The listing builds one solid part. Answer for the finished solid, in the listing's coordinates (mm). Face numbers are marked on the shaded views. Coordinates: 2 decimals unless noted, no trailing zeros. Order: outer loops, then holes, each group sorted by start corner. A loop starts at its lowest first (then second) coordinate and runs counter-clockwise, first axis right, second up.
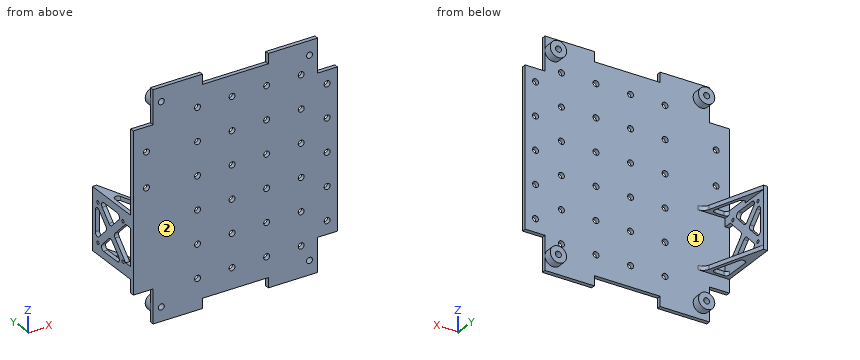
```python
from build123d import *

# Parameters (mm, degrees)
SKETCH1_R            = 2.286
MAIN_BODY_DEPTH      = 3.175
SKETCH34_W           = 7.62
SKETCH34_H           = 50.8
BOSS_EXTRUDE3_DEPTH  = 3.175
SKETCH35_R           = 6.28142
SKETCH35_R_2         = 2.286
BOSS_EXTRUDE4_DEPTH  = 6.35
SKETCH37_W           = 3.175
SKETCH37_H           = 47.625
BOSS_EXTRUDE5_DEPTH  = 45.72
SKETCH40_R           = 1.25
CUT_EXTRUDE3_DEPTH   = 3.175
CUT_EXTRUDE6_REACH   = 188.437
SKETCH48_W           = 28.575
SKETCH48_H           = 6.0825
SKETCH49_R           = 2.286
CUT_EXTRUDE7_DEPTH   = 126.930282399
EXTRUDE_THIN1_DEPTH  = 3.175
FILLET1_R            = 2.54
FILLET2_R            = 6.35
FILLET1_OF_MIRROR2_R = 2.54
FILLET2_OF_MIRROR2_R = 6.35
SKETCH50_R           = 2.286
CUT_EXTRUDE8_DEPTH   = 126.930282399


with BuildPart() as part:
    # Sketch1 → Main Body (new body)
    with BuildSketch(Plane(origin=(0, 0, 0), x_dir=(1, 0, 0), z_dir=(0, 1, 0))):
        Polygon((-25.4, 86.995), (-63.43142, 86.995), (-63.43142, 60.96), (-78.74, 60.96), (-78.74, 25.4), (-71.12, 25.4), (-71.12, -25.4), (-78.74, -25.4), (-78.74, -60.96), (-63.43142, -60.96), (-63.43142, -86.995), (-25.4, -86.995), (-25.4, -79.375), (25.4, -79.375), (25.4, -86.995), (63.43142, -86.995), (63.43142, -60.96), (78.74, -60.96), (78.74, -25.4), (71.12, -25.4), (71.12, 25.4), (78.74, 25.4), (78.74, 60.96), (63.43142, 60.96), (63.43142, 86.995), (25.4, 86.995), (25.4, 79.375), (-25.4, 79.375), align=None)
        with Locations(Location((-57.15, 76.2, 0), (0, 0, 270))):
            Circle(SKETCH1_R, mode=Mode.SUBTRACT)
        with Locations(Location((57.15, 76.2, 0), (0, 0, 270))):
            Circle(SKETCH1_R, mode=Mode.SUBTRACT)
        with Locations(Location((57.15, -76.2, 0), (0, 0, 270))):
            Circle(SKETCH1_R, mode=Mode.SUBTRACT)
        with Locations(Location((-57.15, -76.2, 0), (0, 0, 270))):
            Circle(SKETCH1_R, mode=Mode.SUBTRACT)
    extrude(amount=MAIN_BODY_DEPTH)

    # Sketch34 → Boss-Extrude3 (add)
    with BuildSketch(Plane(origin=(0, 3.175, 0), x_dir=(1, 0, 0), z_dir=(0, 1, 0))):
        with Locations((-74.93, 0)):
            Rectangle(SKETCH34_W, SKETCH34_H)
        with Locations((74.93, 0)):
            Rectangle(SKETCH34_W, SKETCH34_H)
    extrude(amount=-BOSS_EXTRUDE3_DEPTH)

    # Sketch35 → Boss-Extrude4 (add)
    # profile 1 of 4: a face of its own
    with BuildSketch(Plane(origin=(0, 3.175, 0), x_dir=(1, 0, 0), z_dir=(0, 1, 0))):
        with Locations((57.15, 76.2)):
            Circle(SKETCH35_R)
        with Locations(Location((57.15, 76.2, 0), (0, 0, 270))):
            Circle(SKETCH35_R_2, mode=Mode.SUBTRACT)
    # profile 2 of 4: a face of its own
    with BuildSketch(Plane(origin=(0, 3.175, 0), x_dir=(1, 0, 0), z_dir=(0, 1, 0))):
        with Locations((57.15, -76.2)):
            Circle(SKETCH35_R)
        with Locations(Location((57.15, -76.2, 0), (0, 0, 270))):
            Circle(SKETCH35_R_2, mode=Mode.SUBTRACT)
    # profile 3 of 4: a face of its own
    with BuildSketch(Plane(origin=(0, 3.175, 0), x_dir=(1, 0, 0), z_dir=(0, 1, 0))):
        with Locations(Location((-57.15, -76.2, 0), (0, 0, 180))):
            Circle(SKETCH35_R)
        with Locations(Location((-57.15, -76.2, 0), (0, 0, 270))):
            Circle(SKETCH35_R_2, mode=Mode.SUBTRACT)
    # profile 4 of 4: a face of its own
    with BuildSketch(Plane(origin=(0, 3.175, 0), x_dir=(1, 0, 0), z_dir=(0, 1, 0))):
        with Locations(Location((-57.15, 76.2, 0), (0, 0, 180))):
            Circle(SKETCH35_R)
        with Locations(Location((-57.15, 76.2, 0), (0, 0, 270))):
            Circle(SKETCH35_R_2, mode=Mode.SUBTRACT)
    extrude(amount=BOSS_EXTRUDE4_DEPTH)

    # Sketch37 → Boss-Extrude5 (add)
    with BuildSketch(Plane(origin=(0, 3.175, 0), x_dir=(1, 0, 0), z_dir=(0, 1, 0))):
        with Locations((-77.1525, 26.9875)):
            Rectangle(SKETCH37_W, SKETCH37_H)
    extrude(amount=BOSS_EXTRUDE5_DEPTH)

    # Sketch40 → Cut-Extrude3 (cut)
    with BuildSketch(Plane.ZY.offset(78.74)):
        with Locations((-41.9875, 42.355)):
            Circle(SKETCH40_R)
        with Locations((-11.9875, 42.355)):
            Circle(SKETCH40_R)
        with Locations((-11.9875, 12.355)):
            Circle(SKETCH40_R)
        with Locations((-41.9875, 12.355)):
            Circle(SKETCH40_R)
        with BuildLine():
            Line((-35.142897552, 45.4525), (-18.832102448, 45.4525))
            ThreePointArc((-18.832102448, 45.4525), (-16.485448436, 43.884515918), (-17.036051224, 41.116448776))
            Line((-17.036051224, 41.116448776), (-25.191448776, 32.961051224))
            ThreePointArc((-25.191448776, 32.961051224), (-26.9875, 32.217102448), (-28.783551224, 32.961051224))
            Line((-28.783551224, 32.961051224), (-36.938948776, 41.116448776))
            ThreePointArc((-36.938948776, 41.116448776), (-37.489551564, 43.884515918), (-35.142897552, 45.4525))
        make_face()
        with BuildLine():
            Line((-21.381448776, 29.151051224), (-13.226051224, 37.306448776))
            ThreePointArc((-13.226051224, 37.306448776), (-10.457984082, 37.857051564), (-8.89, 35.510397552))
            Line((-8.89, 35.510397552), (-8.89, 19.199602448))
            ThreePointArc((-8.89, 19.199602448), (-10.457984082, 16.852948436), (-13.226051224, 17.403551224))
            Line((-13.226051224, 17.403551224), (-21.381448776, 25.558948776))
            ThreePointArc((-21.381448776, 25.558948776), (-22.125397552, 27.355), (-21.381448776, 29.151051224))
        make_face()
        with BuildLine():
            Line((-25.191448776, 21.748948776), (-12.7, 9.2575))
            Line((-12.7, 9.2575), (-41.275, 9.2575))
            Line((-41.275, 9.2575), (-28.783551224, 21.748948776))
            ThreePointArc((-28.783551224, 21.748948776), (-26.9875, 22.492897552), (-25.191448776, 21.748948776))
        make_face()
        with BuildLine():
            Line((-32.593551224, 25.558948776), (-40.748948776, 17.403551224))
            ThreePointArc((-40.748948776, 17.403551224), (-43.517015918, 16.852948436), (-45.085, 19.199602448))
            Line((-45.085, 19.199602448), (-45.085, 35.510397552))
            ThreePointArc((-45.085, 35.510397552), (-43.517015918, 37.857051564), (-40.748948776, 37.306448776))
            Line((-40.748948776, 37.306448776), (-32.593551224, 29.151051224))
            ThreePointArc((-32.593551224, 29.151051224), (-31.849602448, 27.355), (-32.593551224, 25.558948776))
        make_face()
    extrude(amount=-CUT_EXTRUDE3_DEPTH, mode=Mode.SUBTRACT)

    # Sketch48 → Cut-Extrude6 (cut, up to next)
    with BuildSketch(Plane.ZY.offset(78.74), mode=Mode.PRIVATE) as cut_extrude6_sk1:
        with Locations((-26.9875, 6.21625)):
            Rectangle(SKETCH48_W, SKETCH48_H)
    cut_extrude6_tool1 = extrude(cut_extrude6_sk1.sketch, amount=-CUT_EXTRUDE6_REACH, mode=Mode.PRIVATE) & part.part
    add(cut_extrude6_tool1.solids().sort_by_distance((-78.74, 6.21625, -26.9875))[0], mode=Mode.SUBTRACT)

    # Sketch49 → Cut-Extrude7 (cut, through all)
    with BuildSketch(Plane(origin=(0, 3.175, 0), x_dir=(1, 0, 0), z_dir=(0, 1, 0))):
        with Locations(Location((-68.58, -15.5575, 0), (0, 0, 270))):
            Circle(SKETCH49_R)
        with Locations(Location((-68.58, -42.2275, 0), (0, 0, 270))):
            Circle(SKETCH49_R)
    extrude(amount=-CUT_EXTRUDE7_DEPTH, mode=Mode.SUBTRACT)

    # Sketch39 → Extrude-Thin1 (add)
    with BuildSketch(Plane.XY.offset(-3.175)):
        Polygon((-75.565, 48.895), (-58.924280889, 3.175), (-75.565, 3.175), (-75.565, 5.715), (-62.551776826, 5.715), (-77.951819257, 48.026268836), align=None)
    extrude_thin1 = extrude(amount=-EXTRUDE_THIN1_DEPTH)

    # Fillet1
    fillet1_edges = [part.edges().sort_by_distance(p)[0] for p in [
        (-75.565, 5.715, -4.7625),
        (-75.565, 41.468536824, -4.7625),
        (-62.551776826, 5.715, -4.7625),
    ]]
    fillet(fillet1_edges, radius=FILLET1_R)

    # Fillet2
    fillet2_edges = [part.edges().sort_by_distance(p)[0] for p in [
        (-58.924280889, 3.175, -4.7625),
    ]]
    fillet(fillet2_edges, radius=FILLET2_R)

    # Mirror2: Extrude-Thin1 across plane
    add(extrude_thin1.mirror(Plane(origin=(0, 0, -26.9875), x_dir=(1, 0, 0), z_dir=(0, 0, -1))))

    # Fillet1 of Mirror2
    fillet1_of_mirror2_edges = [part.edges().sort_by_distance(p)[0] for p in [
        (-75.565, 5.715, -49.2125),
        (-75.565, 41.468536824, -49.2125),
        (-62.551776826, 5.715, -49.2125),
    ]]
    fillet(fillet1_of_mirror2_edges, radius=FILLET1_OF_MIRROR2_R)

    # Fillet2 of Mirror2
    fillet2_of_mirror2_edges = [part.edges().sort_by_distance(p)[0] for p in [
        (-58.924280889, 3.175, -49.2125),
    ]]
    fillet(fillet2_of_mirror2_edges, radius=FILLET2_OF_MIRROR2_R)

    # Sketch50 → Cut-Extrude8 (cut, through all)
    with BuildSketch(Plane(origin=(0, 3.175, 0), x_dir=(1, 0, 0), z_dir=(0, 1, 0))):
        with Locations(Location((-29.21, 63.5, 0), (0, 0, 270))):
            Circle(SKETCH50_R)
        with Locations(Location((-2.56286, 63.5, 0), (0, 0, 270))):
            Circle(SKETCH50_R)
        with Locations(Location((24.08428, 63.5, 0), (0, 0, 270))):
            Circle(SKETCH50_R)
        with Locations(Location((50.73142, 63.5, 0), (0, 0, 270))):
            Circle(SKETCH50_R)
        with Locations(Location((-2.56286, 38.1, 0), (0, 0, 270))):
            Circle(SKETCH50_R)
        with Locations(Location((24.08428, 38.1, 0), (0, 0, 270))):
            Circle(SKETCH50_R)
        with Locations(Location((50.73142, 38.1, 0), (0, 0, 270))):
            Circle(SKETCH50_R)
        with Locations(Location((-2.56286, 12.7, 0), (0, 0, 270))):
            Circle(SKETCH50_R)
        with Locations(Location((24.08428, 12.7, 0), (0, 0, 270))):
            Circle(SKETCH50_R)
        with Locations(Location((50.73142, 12.7, 0), (0, 0, 270))):
            Circle(SKETCH50_R)
        with Locations(Location((-2.56286, -12.7, 0), (0, 0, 270))):
            Circle(SKETCH50_R)
        with Locations(Location((24.08428, -12.7, 0), (0, 0, 270))):
            Circle(SKETCH50_R)
        with Locations(Location((50.73142, -12.7, 0), (0, 0, 270))):
            Circle(SKETCH50_R)
        with Locations(Location((-2.56286, -38.1, 0), (0, 0, 270))):
            Circle(SKETCH50_R)
        with Locations(Location((24.08428, -38.1, 0), (0, 0, 270))):
            Circle(SKETCH50_R)
        with Locations(Location((50.73142, -38.1, 0), (0, 0, 270))):
            Circle(SKETCH50_R)
        with Locations(Location((-2.56286, -63.5, 0), (0, 0, 270))):
            Circle(SKETCH50_R)
        with Locations(Location((24.08428, -63.5, 0), (0, 0, 270))):
            Circle(SKETCH50_R)
        with Locations(Location((50.73142, -63.5, 0), (0, 0, 270))):
            Circle(SKETCH50_R)
        with Locations(Location((-29.21, 38.1, 0), (0, 0, 270))):
            Circle(SKETCH50_R)
        with Locations(Location((-29.21, 12.7, 0), (0, 0, 270))):
            Circle(SKETCH50_R)
        with Locations(Location((-29.21, -12.7, 0), (0, 0, 270))):
            Circle(SKETCH50_R)
        with Locations(Location((-29.21, -38.1, 0), (0, 0, 270))):
            Circle(SKETCH50_R)
        with Locations(Location((-29.21, -63.5, 0), (0, 0, 270))):
            Circle(SKETCH50_R)
        with Locations(Location((70.73392, 50.8, 0), (0, 0, 270))):
            Circle(SKETCH50_R)
        with Locations(Location((70.73392, 25.4, 0), (0, 0, 270))):
            Circle(SKETCH50_R)
        with Locations(Location((70.73392, 0, 0), (0, 0, 270))):
            Circle(SKETCH50_R)
        with Locations(Location((70.73392, -25.4, 0), (0, 0, 270))):
            Circle(SKETCH50_R)
        with Locations(Location((70.73392, -50.8, 0), (0, 0, 270))):
            Circle(SKETCH50_R)
    extrude(amount=-CUT_EXTRUDE8_DEPTH, mode=Mode.SUBTRACT)


solid = part.part
```
1) Each of these flat-tipped pins is pushed along its axis until it touches: P1, Ø3.5, axis at x = 24.08, z = 38.1, coming from the -Y side; P2, Ø3.5, axis at x = -71.5, y = 1, coming from the -Z side; P3, Ø5, axis at x = 21.5, z = 26, coming from the +Y side (3 decimals); P4, Ø3.5, axis at y = 1.5, z = -80, coming from the +X side. Where does it stop, or does it pass through?
2) Straight lines are drawn through the part: probe 1 along X at (y, z) = (6.5, -76); probe 2 along X at (y, z) = (2.3, -38.1); probe 3 along X at (y, z) = (2.25, 76.2). For each, find the intervals that lie inside material, in ascending order.
3) A cutting plane is placed at A-A, the plane x = -57.15. Write down the section's boundary in (y, z) (3 decimals), plus the area to 3 significant figures.
4) A cutting plane is placed at C-C, the plane x = 41.5. Write down the section's boundary in (y, z) (3 decimals), plus the area to 3 significant figures.
5) The mould has two halves that part along Z. Classify the marked faces 1 and 2: released by +Z, released by -Z, zero draft, split by the parting line, or undercut.
6) A cutting plane is placed at B-B, the plane x = 13. Write down the section's boundary in (y, z) (3 decimals).
Working result:
1. P1: passes through
1. P2: stops at z = -60.96
1. P3: stops at y = 3.175
1. P4: stops at x = 63.43
2. probe 1: x = -63.43 to -59.43, -54.87 to -50.87, 50.87 to 54.87, 59.43 to 63.43
2. probe 2: x = -78.74 to -31.5, -26.92 to -4.85, -0.28 to 21.8, 26.37 to 48.45, 53.02 to 78.74
2. probe 3: x = -63.43 to -59.44, -54.86 to 54.86, 59.44 to 63.43
3. outline: (0, -86.995) - (3.175, -86.995) - (3.175, -82.481) - (9.525, -82.481) - (9.525, -78.486) - (0, -78.486) - close; (0, -73.914) - (9.525, -73.914) - (9.525, -69.919) - (3.175, -69.919) - (3.175, -50.8) - (3.765, -50.8) - (3.765, -47.625) - (3.175, -47.625) - (3.175, -6.35) - (3.765, -6.35) - (3.765, -3.175) - (3.175, -3.175) - (3.175, 69.919) - (9.525, 69.919) - (9.525, 73.914) - (0, 73.914) - close; (0, 78.486) - (9.525, 78.486) - (9.525, 82.481) - (3.175, 82.481) - (3.175, 86.995) - (0, 86.995) - close
3. area: 629 mm2
4. outline: (0, -86.995) - (3.175, -86.995) - (3.175, 86.995) - (0, 86.995) - close
4. area: 552 mm2
5. face 1: undercut
5. face 2: zero draft
6. outline: (0, -79.375) - (3.175, -79.375) - (3.175, 79.375) - (0, 79.375) - close
